Geometry: final body of the model. Coordinates: model frame, mm. A direction names the side the tool comes from. Round coordinates to 2 decimals unless told otherwise and drop trailing zeros. Loops run counter-clockwise (first coordinate to the right, second up) from the corner with the lowest first, then second, coordinate; pieces in that order, holes last. Notation, with made-up numbers: M 9,5.5 L 38,5.5 A18 ccw 38,19.5 Z; hole C -11,8 d7. An arc over 180 degrees is marked long. Answer as a JSON object with one key per item and string values.
Autodesk Inventor part; units mm, degrees
ref_plane "YZ Plane" through (0, 0, 0) normal (1, 0, 0) x (0, 1, 0)
ref_plane "XZ Plane" through (0, 0, 0) normal (0, 1, 0) x (-1, 0, 0)
ref_plane "XY Plane" through (0, 0, 0) normal (0, 0, 1) x (1, 0, 0)
sketch "Skizze1" plane through (0, 0, 0) normal (0, 0, 1) x (1, 0, 0)
  line L0 (21, 7) -> (-21, 7)
  line L1 (-21, 7) -> (-21, -7)
  line L2 (-21, -7) -> (21, -7)
  line L3 (21, -7) -> (21, 7)
  line L4 (21, 7) -> (-21, -7) construction
  line L5 (-21, 7) -> (21, -7) construction
  point P0 (0, 0)
  dimension "d0" = 42
  dimension "d1" = 14
extrude "Extrusion1" add sketch "Skizze1" along normal blind 6
sketch "Skizze2" plane through (0, 0, 6) normal (0, 0, 1) x (1, 0, 0)
  line L0 (21, 7) -> (-21, 7)
  line L1 (-9, -7) -> (9, -7)
  line L2 (9, -7) -> (9, 7)
  line L3 (9, 7) -> (-9, 7)
  line L4 (-9, 7) -> (-9, -7)
  line L5 (-9, -7) -> (9, 7) construction
  line L6 (9, -7) -> (-9, 7) construction
  point P0 (0, 0)
  dimension "d4" = 18
extrude "Extrusion2" add sketch "Skizze2" along normal blind 26.8
sketch "Skizze3" plane through (-21, -7, 0) normal (0, -1, 0) x (1, 0, 0)
  line L0 (20.8889, 32.8) -> (20.8889, 23.9985)
  line L1 (21.1111, 32.8) -> (21.1111, 23.9985)
  arc A0 (20.8889, 23.9985) -> (21.1111, 23.9985) centre (21, 20) ccw
  line L2 (20.8889, 32.8) -> (21.1111, 32.8)
  line L3 (0, 0) -> (42, 0)
  line L4 (12, 32.8) -> (30, 32.8)
  point P0 (21, 0)
  dimension "d28" = 20
  dimension "d29" = 4
  dimension "d30" = 0
extrude "Extrusion3" cut sketch "Skizze3" against normal through all
sketch "Skizze4" plane through (9, -7, 6) normal (1, 0, 0) x (0, 0, -1)
  circle A0 centre (-22.3, 7) radius 2.25
  line L0 (-26.8, 0) -> (-26.8, 14)
  point P0 (6, 7)
  dimension "d13" = 4.5
  dimension "d31" = 4.5
extrude "Extrusion4" cut sketch "Skizze4" against normal through all
sketch "Skizze5" plane through (9, -7, 6) normal (1, 0, 0) x (0, 0, -1)
  circle A0 centre (-22.3, 7) radius 2.25
  circle A1 centre (-22.3, 7) radius 3.75
  point P0 (6, 7)
  dimension "d16" = 7.5
extrude "Extrusion5" cut sketch "Skizze5" against normal blind 3.5
sketch "Skizze6" plane through (0, 0, 6) normal (0, 0, 1) x (1, 0, 0)
  circle A0 centre (16, 0) radius 2.75
  circle A1 centre (-16, 0) radius 2.75
  line L0 (-21, 7) -> (-21, -7)
  point P0 (0, 0)
  dimension "d19" = 5.5
  dimension "d20" = 5.5
  dimension "d21" = 32
  dimension "d22" = 5
extrude "Extrusion6" cut sketch "Skizze6" against normal up to next
chamfer "Fase1" distance 0.5 angle 45 14 edges at (21, 0, 6) (-21, 0, 6) (15, 7, 6) (-15, 7, 6) (-15, -7, 6) (15, -7, 6) (9, 0, 32.8) (-9, 0, 32.8) (-4.5556, -7, 32.8) (4.5556, -7, 32.8) (4.5556, 7, 32.8) (-4.5556, 7, 32.8) (13.25, 0, 6) (-18.75, 0, 6)
properties part number "SK12" material "Aluminium 5005"
1) Section query B-B (x = 2.5). Return the cut outline in (y, z).
Results:
{"outline": "M -7,0 L 7,0 L 7,16.88 L -7,16.88 Z; M -7,23.12 L 7,23.12 L 7,32.3 L 6.5,32.8 L -6.5,32.8 L -7,32.3 Z; hole C 0,28.3 d4.5"}
2) Reachability of faces 1 (the flat face through (-21, 0, 3)), 2 (the flat face through (5.5, 0.1, 25.9)), 3 (the flat face through (12, 0, 6)), 4 (the flat face through (0, 7, 12)), 5 (the flat face through (-12, 0, 6)) from +Z, -Z, +X, -X, +Y, -Y: full face, straight path, thin tool, end or side. Return the list, or none.
Results:
{"face 1": "+Z, -Z, -X, +Y, -Y", "face 2": "+X", "face 3": "+Z, +X, +Y, -Y", "face 4": "+Z, -Z, +X, -X, +Y", "face 5": "+Z, -X, +Y, -Y"}
3) Ray query, line 1 (Y direction, x = 16, z = 2); line 2 (Y direction, x = 2.65, z = 28.3); line 3 (X direction, y = 2, z = 30). Return the intervals inside material, ascending.
Results:
{"line 1": "-7 to -2.75, 2.75 to 7", "line 2": "-7 to -2.25, 2.25 to 7", "line 3": "-9 to -0.11, 0.11 to 5.5"}
4) Pull-direction query (X, two-part tool) for faces 6 (the flat face through (21, 0, 3)), 7 (the cylindrical face through (-4.49, 1.52, 29.96)), 8 (the flat face through (0.111, -1.7, 26.5)); classes: +X half, -X half, draft (parallel to the pull), parting line (faces both ways), or undercut.
Results:
{"face 6": "+X half", "face 7": "draft", "face 8": "undercut"}
5) Pin query (flat end, axial travel): P1, Ø3.5, axis at x = 14, y = 2, coming from the +Z side; P2, Ø6, axis at y = 0, z = 28.3, coming from the +X side; P3, Ø7, axis at y = -3, z = 17.5, coming from the +X side. Return the tip coordinate at first contact, or that it passes through.
Results:
{"P1": "z = 6", "P2": "x = 5.5", "P3": "x = 9"}
6) Section query C-C (x = 16). Return the cut outline in (y, z).
Results:
{"outline": "M -7,0 L -2.75,0 L -2.75,5.5 L -3.25,6 L -6.5,6 L -7,5.5 Z; M 2.75,0 L 7,0 L 7,5.5 L 6.5,6 L 3.25,6 L 2.75,5.5 Z"}
7) Section query A-A (z = 28.3). Return the cut outline in (x, y).
Results:
{"outline": "M -9,-7 L -0.11,-7 L -0.11,-2.25 L -9,-2.25 Z; M -9,2.25 L -0.11,2.25 L -0.11,7 L -9,7 Z; M 0.11,-7 L 9,-7 L 9,-3.75 L 5.5,-3.75 L 5.5,-2.25 L 0.11,-2.25 Z; M 0.11,2.25 L 5.5,2.25 L 5.5,3.75 L 9,3.75 L 9,7 L 0.11,7 Z"}
8) Section query D-D (y = 0). Count the separate pieces of the cut face and the enclosed holes in it, and give its area (3 significant figures).
Results:
{"separate pieces": "5", "enclosed holes": "0", "area": "525 mm2"}
